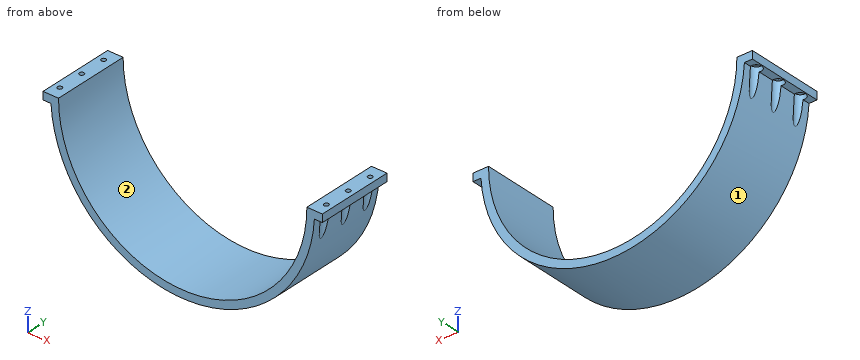
```python
from build123d import *

# Parameters (mm, degrees)
BOSS_EXTRUDE1_DEPTH     = 50
SKETCH2_W               = 5
SKETCH2_H               = 50
BOSS_EXTRUDE2_DEPTH     = 5
BOSS_EXTRUDE2_2_DEPTH   = 5
SKETCH3_W               = 8.095126166
SKETCH3_H               = 5
BOSS_EXTRUDE3_DEPTH     = 50
CUT_EXTRUDE1_DEPTH      = 131.384048104
CUT_EXTRUDE1_DEPTH_BACK = 3
SKETCH4_R               = 3.5
SKETCH5_R               = 1.5
CUT_EXTRUDE2_DEPTH      = 133.245983026


with BuildPart() as part:
    # Sketch1 → Boss-Extrude1 (new body)
    with BuildSketch(Plane(origin=(0, 0, 0), x_dir=(1, 0, 0), z_dir=(0, 1, 0))):
        with BuildLine():
            Line((-85, 0), (-80, 0))
            ThreePointArc((-80, 0), (0, 80), (80, 0))
            Line((80, 0), (85, 0))
            ThreePointArc((85, 0), (0, 85), (-85, 0))
        make_face()
    extrude(amount=BOSS_EXTRUDE1_DEPTH)



with BuildPart() as body_2:
    # Sketch2 → Boss-Extrude2 (new body)
    with BuildSketch(Plane.XY):
        with Locations((87.5, 25)):
            Rectangle(SKETCH2_W, SKETCH2_H)
    extrude(amount=-BOSS_EXTRUDE2_DEPTH)


with BuildPart() as body_3:
    # Sketch2 → Boss-Extrude2 2 (new body)
    with BuildSketch(Plane.XY):
        with Locations((-87.5, 25)):
            Rectangle(SKETCH2_W, SKETCH2_H)
    extrude(amount=-BOSS_EXTRUDE2_2_DEPTH)


with BuildPart() as part_1:
    add(part.part)

    add(body_2.part)  # Boss-Extrude3 merges body 2

    add(body_3.part)  # Boss-Extrude3 merges body 3
    # Sketch3 → Boss-Extrude3 (add)
    with BuildSketch(Plane(origin=(0, 50, 0), x_dir=(1, 0, 0), z_dir=(0, 1, 0))):
        with Locations((-85.952436917, 2.5)):
            Rectangle(SKETCH3_W, SKETCH3_H)
        with Locations((85.952436917, 2.5)):
            Rectangle(SKETCH3_W, SKETCH3_H)
    extrude(amount=-BOSS_EXTRUDE3_DEPTH)

    # Sketch4 → Cut-Extrude1 (cut, two sides: drawn at the far end of the back side and taken through both)
    with BuildSketch(Plane(origin=(0, 0, -5), x_dir=(-1, 0, 0), z_dir=(0, 0, -1)).offset(-CUT_EXTRUDE1_DEPTH_BACK)):
        with Locations(Location((85.852813742, 42, 0), (0, 0, 253.398450401))):
            Circle(SKETCH4_R)
        with Locations(Location((85.852813742, 25, 0), (0, 0, 253.398450401))):
            Circle(SKETCH4_R)
        with Locations(Location((85.852813742, 8, 0), (0, 0, 253.398450401))):
            Circle(SKETCH4_R)
        with Locations(Location((-85.852813742, 8, 0), (0, 0, 180))):
            Circle(SKETCH4_R)
        with Locations(Location((-85.852813742, 25, 0), (0, 0, 180))):
            Circle(SKETCH4_R)
        with Locations(Location((-85.852813742, 42, 0), (0, 0, 180))):
            Circle(SKETCH4_R)
    extrude(amount=CUT_EXTRUDE1_DEPTH + CUT_EXTRUDE1_DEPTH_BACK, mode=Mode.SUBTRACT)

    # Sketch5 → Cut-Extrude2 (cut, through all)
    with BuildSketch(Plane(origin=(0, 0, -2), x_dir=(-1, 0, 0), z_dir=(0, 0, -1))):
        with Locations((85.852813742, 42)):
            Circle(SKETCH5_R)
        with Locations((85.852813742, 25)):
            Circle(SKETCH5_R)
        with Locations(Location((-85.852813742, 8, 0), (0, 0, 180))):
            Circle(SKETCH5_R)
        with Locations((85.852813742, 8)):
            Circle(SKETCH5_R)
        with Locations(Location((-85.852813742, 25, 0), (0, 0, 180))):
            Circle(SKETCH5_R)
        with Locations(Location((-85.852813742, 42, 0), (0, 0, 180))):
            Circle(SKETCH5_R)
    extrude(amount=-CUT_EXTRUDE2_DEPTH, mode=Mode.SUBTRACT)


solid = part_1.part
```
Can you work these out from the model? Positions are in its coordinate system, mm. Face numbers are marked on the shaded views. Coordinates: 2 decimals unless noted, no trailing zeros. Loops run counter-clockwise (first coordinate to the right, second up) from the corner with the lowest first, then second, coordinate; pieces in that order, holes last. Notation, with made-up numbers: (-36.5, -7.75) - (3.5, -7.75) arc R16 cw to (3.5, 19.25) - close; hole circle Ø6 at (52, -9). An arc over 180 degrees is marked (long way). Use a Markdown table: item, result.
Item 1: If I drill on probe 1 along X at (y, z) = (8, -13); probe 2 along X at (y, z) = (24.5, -34); probe 3 along Z at (x, y) = (34.5, 41), over which ranges is the centre line in solid material (lowest first)? Write a range as from..to.
Numbers:
| item | result |
|---|---|
| probe 1 | x = -82.35..-78.94, 78.94..82.35 |
| probe 2 | x = -77.9..-72.42, 72.42..77.9 |
| probe 3 | z = -77.68..-72.18 |
Item 2: Will these pins go through, and if not, where does the flat tip stop? pin 1 (8 mm diameter, centred on y = 14, z = -11.5, fed in from +X); pin 2 (3 mm diameter, centred on x = 7, y = 22, fed in from -Z); pin 3 (3.5 mm diameter, centred on x = -85.85, y = 25, fed in from -Z).
Numbers:
| item | result |
|---|---|
| pin 1 | stops at x = 84.67 |
| pin 2 | stops at z = -84.82 |
| pin 3 | stops at z = -2 |
Item 3: I want a section at D-D on x = 0. Please give me the cut outline in (y, z).
Numbers:
| item | result |
|---|---|
| outline | (0, -85) - (50, -85) - (50, -80) - (0, -80) - close |
Item 4: We'd pull the mould along X, two halves only. Please class the marked faces 1 and 2: released by +X, released by -X, zero draft, split by the parting line, or undercut.
Numbers:
| item | result |
|---|---|
| face 1 | split by the parting line |
| face 2 | undercut |
Item 5: I want a section at C-C on z = -62. Please give me the cut outline in (x, y).
Numbers:
| item | result |
|---|---|
| outline | (-58.15, 0) - (-50.56, 0) - (-50.56, 50) - (-58.15, 50) - close; (50.56, 0) - (58.15, 0) - (58.15, 50) - (50.56, 50) - close |
Item 6: I want a section at B-B on y = 17. Please give me the cut outline in (x, z), and give its area (3 significant figures).
Numbers:
| item | result |
|---|---|
| outline | (-90, -5) - (-84.85, -5) arc R85 ccw to (84.85, -5) - (90, -5) - (90, 0) - (80, 0) arc R80 cw to (-80, 0) - (-90, 0) - close |
| area | 1,350 mm2 |
Item 7: I want a section at A-A on z = -7. Please give me the cut outline in (x, y), and give its area (3 significant figures).
Numbers:
| item | result |
|---|---|
| outline | (-84.71, 0) - (-79.69, 0) - (-79.69, 50) - (-84.71, 50) - (-84.71, 45.31) arc R3.5 cw to (-84.71, 38.69) - (-84.71, 28.31) arc R3.5 cw to (-84.71, 21.69) - (-84.71, 11.31) arc R3.5 cw to (-84.71, 4.69) - close; (79.69, 0) - (84.71, 0) - (84.71, 4.69) arc R3.5 cw to (84.71, 11.31) - (84.71, 21.69) arc R3.5 cw to (84.71, 28.31) - (84.71, 38.69) arc R3.5 cw to (84.71, 45.31) - (84.71, 50) - (79.69, 50) - close |
| area | 433 mm2 |
